Work out the finished part from the listing and answer in its coordinate system (mm). Coordinates: 2 decimals unless noted, no trailing zeros. Write each loop counter-clockwise with the first axis right and the second up, starting at its lowest first coordinate (ties: lowest second). Pieces come first, ordered by that corner, then holes. Notation, with made-up numbers: (63.25, 36.5) - (102.25, 36.5) arc R23 ccw to (102.25, 61.5) - close; hole circle Ø5 at (-23, 77.25). An arc over 180 degrees is marked (long way). Answer as a JSON object with one key per item and string values. Group by question number.
Autodesk Inventor part; units mm, degrees
ref_plane "YZ Plane" through (0, 0, 0) normal (1, 0, 0) x (0, 1, 0)
ref_plane "XZ Plane" through (0, 0, 0) normal (0, 1, 0) x (-1, 0, 0)
ref_plane "XY Plane" through (0, 0, 0) normal (0, 0, 1) x (1, 0, 0)
sketch "Sketch1" plane through (0, 0, 0) normal (0, 0, 1) x (1, 0, 0)
  circle A0 centre (0, 0) radius 20
  circle A1 centre (0, 0) radius 18
  dimension "d0" = 40
  dimension "d1" = 2
extrude "Extrusion1" add sketch "Sketch1" along normal blind 1000
chamfer "Chamfer1" distance 1 angle 45 1 edges at (-20, 0, 1000)
chamfer "Chamfer2" distance 1 angle 45 1 edges at (-20, 0, 0)
properties part number "STK00-001" material "Polypropylene"
Q1. Section A-A on x = 0 is taken. Determine the outline of the cut face in (y, z).
Q2. Section C-C on z = 933.5 is taken. Determine the outline of the cut face in (x, y), plus the area to 3 significant figures.
Q3. Consider L1, parallel to Y at x = 0.5, z = 585; L2, parallel to Y at x = 3.5, z = 399; L3, parallel to Z at x = -11, y = 15.5. Determine where each line is inside the solid, lowest interval first. Write a range as from..to.
Q4. Flat-ended cylindrical pins translate along their axes: pin 1 Ø10 at (x, y) = (14, 3) entering from -Z; pin 2 Ø8 at (x, z) = (-11.5, 238.5) entering from -Y; pin 3 Ø2 at (x, z) = (15.5, 866) entering from +Y (3 decimals); pin 4 Ø3 at (y, z) = (-7.5, 681.5) entering from -X. Find the tip coordinate at first contact, or state that the pin passes through.
Numbers:
{
 "1": {"outline": "(-20, 1) - (-19, 0) - (-18, 0) - (-18, 1000) - (-19, 1000) - (-20, 999) - close; (18, 0) - (19, 0) - (20, 1) - (20, 999) - (19, 1000) - (18, 1000) - close"},
 "2": {"outline": "circle Ø40 at (0, 0); hole circle Ø36 at (0, 0)", "area": "239 mm²"},
 "3": {"L1": "y = -19.99..-17.99, 17.99..19.99", "L2": "y = -19.69..-17.66, 17.66..19.69", "L3": "z = 0.01..999.99"},
 "4": {"pin 1": "stops at z = 0", "pin 2": "stops at y = -18.54", "pin 3": "stops at y = 13.775", "pin 4": "stops at x = -19.08"}
}
